Verification items for the finished model (mm, model axes). A direction names the side the tool comes from. Coordinates: 2 decimals unless noted, no trailing zeros. Order: outer loops, then holes, each group sorted by start corner. A loop starts at its lowest first (then second) coordinate and runs counter-clockwise, first axis right, second up. Notation, with made-up numbers: (34.25, -25.75) - (68.25, -25.75) arc R20 ccw to (68.25, 6.25) - close; hole circle Ø4 at (79.25, 26). An arc over 180 degrees is marked (long way). Answer as CSV lines item,"result". Start each with the question number.
1. Section check C-C (z = 2.75). Record the cut outline in (x, y), and give its area (3 significant figures).
2. Mould release check, pull along Y, two halves, no side actions. Record for faces 1 (the flat face through (-8.5, -1, 3)), 2 (the flat face through (2.5, -1, 3)), 3 (the flat face through (-2.5, -1, 3)), 4 (the flat face through (0, 5, 3)): pulls with the +Y half, pulls with the -Y half, needs draft (parallel to the pull), parting line crosses it, or undercut.
3. Section check B-B (x = -6). Record the cut outline in (y, z), and give its area (3 significant figures).
4. Section check A-A (y = -2). Record the cut outline in (x, z).
5. Go/stop test with flat-tipped pins: pin 1 (6.5 mm diameter, centred on x = -0.5, y = 0, fed in from +Z); pin 2 (2.5 mm diameter, centred on x = 6, y = -2, fed in from +Z). Record where each tip stops, or that it passes through.
6. Material ranges on L1, parallel to X at y = -3.75, z = 6; L2, parallel to Y at x = 6, z = 2; L3, parallel to Y at x = 1.25, z = 6, recorded low to high. Write a range as [from, to].
7. Section check D-D (y = 3.75). Record the cut outline in (x, z).
8. Set-up check for faces 5 (the flat face through (-1.8, -1, 3)), 6 (the flat face through (6, 0, 7)), 7 (the flat face through (-2, 0, 6.4)): record each of +Z, -Z, +X, -X, +Y, -Y from which the full face is reachable in a straight line by a thin tool's end or side.
Autodesk Inventor part; units mm, degrees
ref_plane "YZ Plane" through (0, 0, 0) normal (1, 0, 0) x (0, 1, 0)
ref_plane "XZ Plane" through (0, 0, 0) normal (0, 1, 0) x (-1, 0, 0)
ref_plane "XY Plane" through (0, 0, 0) normal (0, 0, 1) x (1, 0, 0)
sketch "スケッチ1" plane through (0, 0, 0) normal (0, 0, 1) x (1, 0, 0)
  line L0 (8.5, 7) -> (-8.5, 7)
  line L1 (-8.5, 7) -> (-8.5, -7)
  line L2 (-8.5, -7) -> (8.5, -7)
  line L3 (8.5, -7) -> (8.5, 7)
  line L4 (8.5, 7) -> (-8.5, -7) construction
  line L5 (-8.5, 7) -> (8.5, -7) construction
  circle A0 centre (-6, -2) radius 1.5
  circle A1 centre (6, -2) radius 1.5
  line L6 (-8.5, -6) -> (8.5, -6)
  line L7 (-8.5, 3.5) -> (8.5, 3.5)
  line L8 (-4, -7) -> (-4, 7)
  line L9 (4, -7) -> (4, 7)
  line L10 (2.5, -6) -> (2.5, 3.5)
  line L11 (-2.5, -6) -> (-2.5, 3.5)
  line L12 (1.8, -6) -> (1.8, 3.5)
  line L13 (-1.8, -6) -> (-1.8, 3.5)
  point P0 (0, 0)
  point P1 (-4, -6)
  point P2 (-4, 3.5)
  point P3 (4, -6)
  point P4 (4, 3.5)
  dimension "d0" = 17
  dimension "d1" = 14
  dimension "d2" = 3
  dimension "d3" = 3
  dimension "d4" = 3.5
  dimension "d5" = 4.5
  dimension "d6" = 4.5
  dimension "d7" = 1.5
  dimension "d8" = 1.5
  dimension "d9" = 1
  dimension "d16" = 0.7
  dimension "d17" = 0.7
  dimension "d22" = 5
  dimension "d23" = 5
extrude "押し出し1" add sketch "スケッチ1" along normal blind 7 contours L3 L7 L9 L0 | L9 L7 L8 L0 | L3 L6 L9 L7 | L8 L7 L1 L0 | L3 L2 L9 L6 | L8 L6 L1 L7 | L10 L6 L12 L7 | L9 L2 L8 L6 | L7 L13 L6 L11 | L8 L2 L1 L6
sketch "スケッチ2" plane through (0, 0, 7) normal (0, 0, 1) x (1, 0, 0)
  line L0 (8.5, 7) -> (-8.5, 7)
  line L1 (0, 7) -> (-4, 7)
  line L2 (-4, 7) -> (-4, -7)
  line L3 (-8.5, -7) -> (8.5, -7)
  line L4 (-4, -7) -> (4, -7)
  line L5 (4, -7) -> (4, 7)
  line L6 (4, 7) -> (0, 7)
  point P0 (0, 0)
  dimension "d12" = 4
  dimension "d13" = 8
extrude "押し出し2" cut sketch "スケッチ2" against normal blind 0.6
sketch "スケッチ3" plane through (-8.5, 7, 0) normal (0, 1, 0) x (1, 0, 0)
  line L0 (0, 0) -> (0, -7)
  line L1 (17, 0) -> (17, -7)
  line L2 (0, 0) -> (17, 0)
  line L3 (17, 0) -> (17, -7)
  line L4 (17, -7) -> (0, -7)
  line L5 (0, -7) -> (0, 0)
  point P0 (8.5, 0)
  point P1 (0, -7)
extrude "押し出し3" cut sketch "スケッチ3" against normal blind 2
properties part number "greiper_TPU" material "ゴム、シリコーン"
Evaluation:
1,outline,"(-8.5, -7) - (8.5, -7) - (8.5, 5) - (-8.5, 5) - close; hole circle Ø3 at (-6, -2); hole (-4, -6) - (-2.5, -6) - (-2.5, 3.5) - (-4, 3.5) - close; hole (-1.8, -6) - (1.8, -6) - (1.8, 3.5) - (-1.8, 3.5) - close; hole (2.5, -6) - (4, -6) - (4, 3.5) - (2.5, 3.5) - close; hole circle Ø3 at (6, -2)"
1,area,"127 mm²"
2,face 1,"needs draft"
2,face 2,"undercut"
2,face 3,"undercut"
2,face 4,"pulls with the +Y half"
3,outline,"(-7, 0) - (-3.5, 0) - (-3.5, 7) - (-7, 7) - close; (-0.5, 0) - (5, 0) - (5, 7) - (-0.5, 7) - close"
3,area,"63.0 mm²"
4,outline,"(-8.5, 0) - (-7.5, 0) - (-7.5, 7) - (-8.5, 7) - close; (-4.5, 0) - (-4, 0) - (-4, 7) - (-4.5, 7) - close; (-2.5, 0) - (-1.8, 0) - (-1.8, 6.4) - (-2.5, 6.4) - close; (1.8, 0) - (2.5, 0) - (2.5, 6.4) - (1.8, 6.4) - close; (4, 0) - (4.5, 0) - (4.5, 7) - (4, 7) - close; (7.5, 0) - (8.5, 0) - (8.5, 7) - (7.5, 7) - close"
5,pin 1,"stops at z = 6.4"
5,pin 2,"passes through"
6,L1,"x = [-8.5, -4], [-2.5, -1.8], [1.8, 2.5], [4, 8.5]"
6,L2,"y = [-7, -3.5], [-0.5, 5]"
6,L3,"y = [-7, -6], [3.5, 5]"
7,outline,"(-8.5, 0) - (8.5, 0) - (8.5, 7) - (4, 7) - (4, 6.4) - (-4, 6.4) - (-4, 7) - (-8.5, 7) - close"
8,face 5,"+Z, -Z"
8,face 6,"+Z, +X, -X, +Y, -Y"
8,face 7,"+Z, +Y, -Y"
